The drawing under review shows one solid part. Ordinate dimensions are in mm from its lowest x, y, z. A direction names the side the tool comes from. Give positions to 0.01 mm unless a question says otherwise; leave off trailing zeros. Order: outer loops, then holes, each group sorted by start corner. A loop starts at its lowest first (then second) coordinate and runs counter-clockwise, first axis right, second up. Notation, with made-up numbers: (32.25, 2.25) - (45.25, 2.25) arc R29 ccw to (45.25, 34.25) - close; hole circle Ø8 at (6.5, 23.25). An arc over 180 degrees is marked (long way). Write item = value, one per line. Start each with the question number.
1. We need section D-D, the plane x = 28. Give the boundary of the cut face in (y, z), and give its area (3 significant figures).
2. We need section C-C, the plane z = 15. Give the boundary of the cut face in (x, y) (3 decimals).
3. We need section A-A, the plane y = 2.75. Give the boundary of the cut face in (x, z) (3 decimals).
4. For P1, Ø3.5, axis at y = 4.5, z = 1.5, coming from the -X side; P2, Ø5, axis at y = 9, z = 1.5, coming from the +X side; P3, Ø7, axis at y = 6.5, z = 6.5, coming from the -X side; P4, Ø6, axis at y = 8.5, z = 15, coming from the -X side, all flat-tipped, find the tip position at first contact; note any pin that passes through.
5. Mouldability with a two-part tool opening along Z and no side actions: class the marked faces 4, 5, 6 and 7 as pulls with the +Z half, pulls with the -Z half, needs draft (parallel to the pull), parting line crosses it, or undercut.
6. We need section B-B, the plane x = 14.5. Give the boundary of the cut face in (y, z) (3 decimals), and give its area (3 significant figures).
7. Machinability: for the marked faces 1, 2 and 3, which of the approach directions +Z, -Z, +X, -X, +Y, -Y give a long, thin tool a straight path to every point of the face, cutting with its end or side? Answer none if there is none.
8. Wall thickness on probe 1 along X at (y, z) = (2.25, 8.5); probe 2 along X at (y, z) = (2.25, 13.75); probe 3 along Z at (x, y) = (30, 0.75): over which ranges is each line inside the solid? List them lowest first.
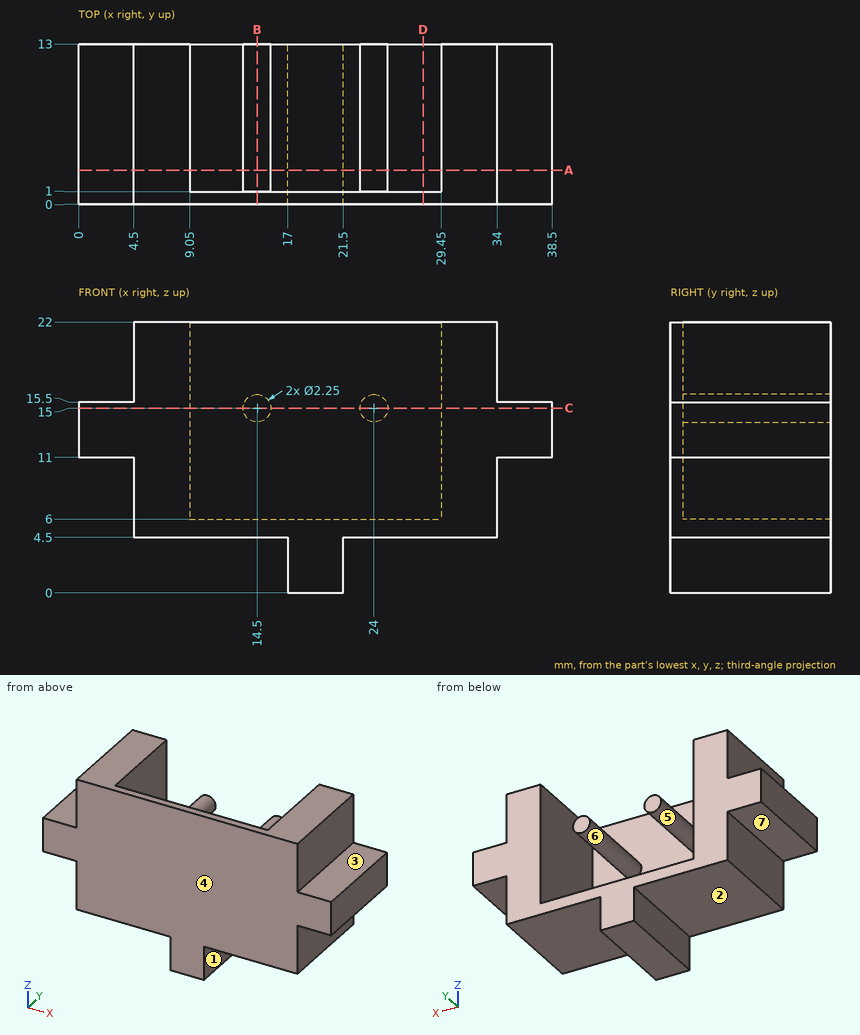
Model answer:
q1.outline = (0, 4.5) - (13, 4.5) - (13, 6) - (1, 6) - (1, 22) - (0, 22) - close
q1.area = 35.5 mm2
q2.outline = (0, 0) - (38.5, 0) - (38.5, 13) - (29.45, 13) - (29.45, 1) - (25.125, 1) - (25.125, 13) - (22.875, 13) - (22.875, 1) - (15.625, 1) - (15.625, 13) - (13.375, 13) - (13.375, 1) - (9.05, 1) - (9.05, 13) - (0, 13) - close
q3.outline = (0, 11) - (4.5, 11) - (4.5, 4.5) - (17, 4.5) - (17, 0) - (21.5, 0) - (21.5, 4.5) - (34, 4.5) - (34, 11) - (38.5, 11) - (38.5, 15.5) - (34, 15.5) - (34, 22) - (29.45, 22) - (29.45, 6) - (9.05, 6) - (9.05, 22) - (4.5, 22) - (4.5, 15.5) - (0, 15.5) - close; circle Ø2.25 at (14.5, 15); circle Ø2.25 at (24, 15)
q4.P1 = 17
q4.P2 = 21.5
q4.P3 = 4.5
q4.P4 = 0
q5.face_4 = needs draft
q5.face_5 = undercut
q5.face_6 = undercut
q5.face_7 = pulls with the -Z half
q6.outline = (0, 4.5) - (13, 4.5) - (13, 6) - (1, 6) - (1, 13.875) - (13, 13.875) - (13, 16.125) - (1, 16.125) - (1, 22) - (0, 22) - close
q6.area = 62.5 mm2
q7.face_1 = -Z, +X, +Y, -Y
q7.face_2 = -Z, -X, +Y, -Y
q7.face_3 = +Z, +X, +Y, -Y
q8.probe_1 = 4.5 to 9.05, 29.45 to 34
q8.probe_2 = 0 to 9.05, 29.45 to 38.5
q8.probe_3 = 4.5 to 22
